Job drawing, mm, ordinate dimensions from the low corner. One solid piece. A direction names the side the tool comes from. Give positions to 0.01 mm unless a question says otherwise; leave off trailing zeros. Order: outer loops, then holes, each group sorted by start corner. A loop starts at its lowest first (then second) coordinate and runs counter-clockwise, first axis right, second up. Notation, with made-up numbers: (-35.5, 85.25) - (-2.5, 85.25) arc R37 cw to (-2.5, 124.25) - close; hole circle Ø8 at (63, 17). An arc over 180 degrees is marked (long way). One line per item, written item: value.
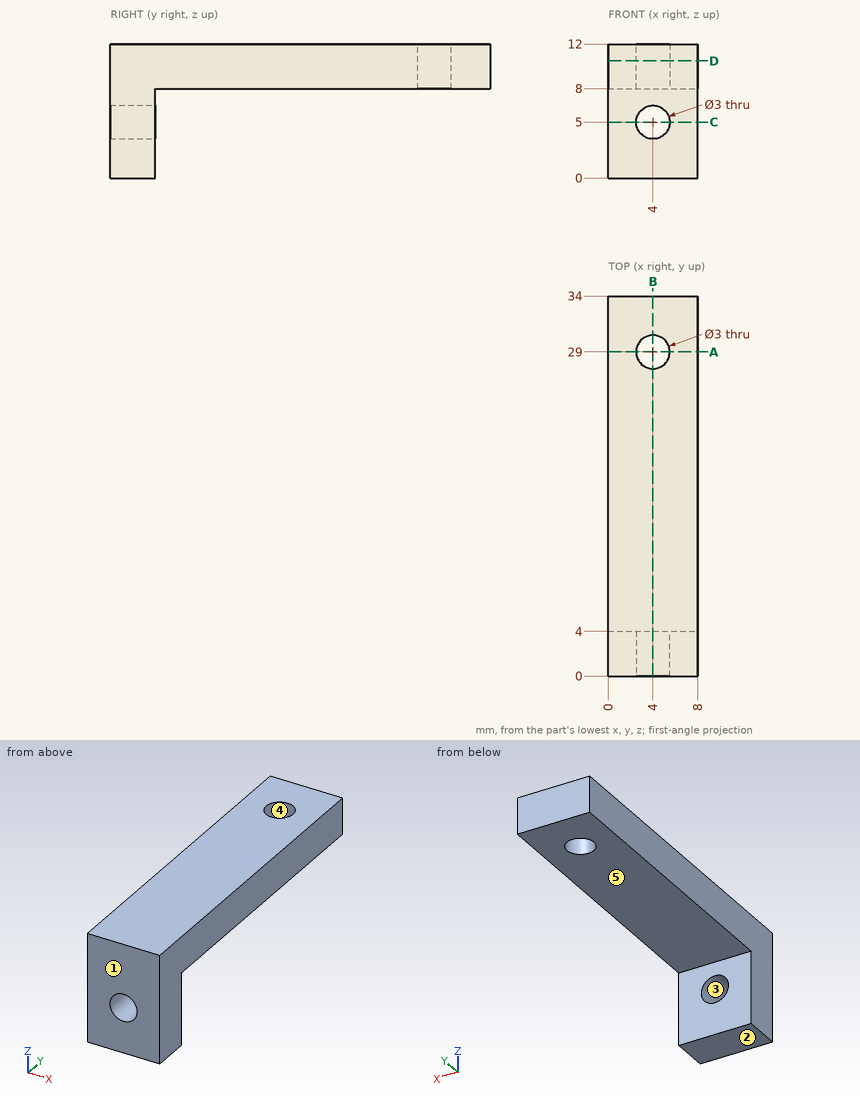
1) Wall check: line 1 along Y through (x, z) = (4, 9.6); line 2 along Z through (x, y) = (4, 3.2); line 3 along Z through (x, y) = (6.75, 14). Give the ranges that are in metal, low to high. Write a range as [from, to].
Answer:
line 1: y = [0, 27.5], [30.5, 34]
line 2: z = [0, 3.5], [6.5, 12]
line 3: z = [8, 12]
2) Slice it at A-A on y = 29. Write the cut outline in (x, z).
Answer:
outline: (0, 8) - (2.5, 8) - (2.5, 12) - (0, 12) - close; (5.5, 8) - (8, 8) - (8, 12) - (5.5, 12) - close
3) Drop a flat-ended pin along its axis: P1, Ø2.5, axis at x = 4, y = 19.5, coming from the -Z side. Give the stop position or say it passes through.
Answer:
P1: stops at z = 8
4) Slice it at B-B on x = 4. Write the cut outline in (y, z), then the cut area to 3 significant figures.
Answer:
outline: (0, 0) - (4, 0) - (4, 3.5) - (0, 3.5) - close; (0, 6.5) - (4, 6.5) - (4, 8) - (27.5, 8) - (27.5, 12) - (0, 12) - close; (30.5, 8) - (34, 8) - (34, 12) - (30.5, 12) - close
area: 144 mm2
5) Slice it at C-C on z = 5. Write the cut outline in (x, y), then the cut area to 3 significant figures.
Answer:
outline: (0, 0) - (2.5, 0) - (2.5, 4) - (0, 4) - close; (5.5, 0) - (8, 0) - (8, 4) - (5.5, 4) - close
area: 20.0 mm2
6) Which spindle directions (+Z, -Z, +X, -X, +Y, -Y) get a long thin tool onto all of the face, cutting with end or side? Do the marked faces 4 and 5. Say none if no direction does.
Answer:
face 4: +Z, -Z
face 5: -Z, +X, -X, +Y
7) Two-plate mould, pull along Z, no slides. Class the marked faces 1, 2 and 3: pulls with the +Z half, pulls with the -Z half, needs draft (parallel to the pull), parting line crosses it, or undercut.
Answer:
face 1: needs draft
face 2: pulls with the -Z half
face 3: undercut
8) Slice it at D-D on z = 10.5. Write the cut outline in (x, y), then the cut area to 3 significant figures.
Answer:
outline: (0, 0) - (8, 0) - (8, 34) - (0, 34) - close; hole circle Ø3 at (4, 29)
area: 265 mm2
